Print and shaded views of the part. All mm, measured from the part's lowest x, y and z. Give positions to 0.01 mm unless a question says otherwise; leave off trailing zeros. Loops run counter-clockwise (first coordinate to the right, second up) from the corner with the lowest first, then second, coordinate; pieces in that order, holes last. Notation, with made-up numbers: (13.25, 68.5) - (55.25, 68.5) arc R21 cw to (55.25, 80.5) - close; hole circle Ø11 at (3.25, 74). An arc over 180 degrees is marked (long way). Return JSON: item names as keys, results as strings.
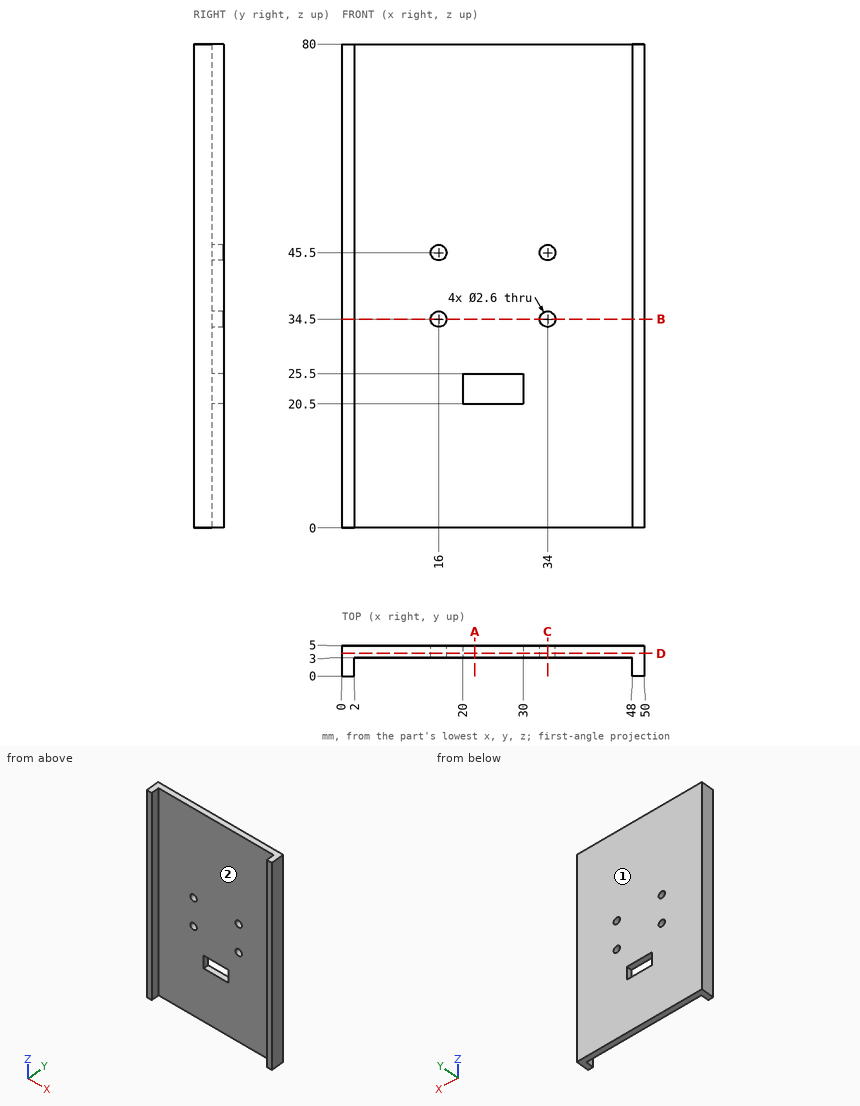
1. Cut at B-B, the plane z = 34.5. Write the cut outline in (x, y).
Values follow:
{"outline": "(0, 0) - (2, 0) - (2, 3) - (14.7, 3) - (14.7, 5) - (0, 5) - close; (17.3, 3) - (32.7, 3) - (32.7, 5) - (17.3, 5) - close; (35.3, 3) - (48, 3) - (48, 0) - (50, 0) - (50, 5) - (35.3, 5) - close"}
2. Cut at C-C, the plane x = 34. Write the cut outline in (y, z), plus the area to 3 significant figures.
Values follow:
{"outline": "(3, 0) - (5, 0) - (5, 33.2) - (3, 33.2) - close; (3, 35.8) - (5, 35.8) - (5, 44.2) - (3, 44.2) - close; (3, 46.8) - (5, 46.8) - (5, 80) - (3, 80) - close", "area": "150 mm²"}
3. Drill centre lines: probe 1 along Z at (x, y) = (34, 4.55); probe 2 along X at (y, z) = (4, 45.5); probe 3 along Z at (x, y) = (21, 4.3). Where is each one in solid material? Low to high.
Values follow:
{"probe 1": "z = 0 to 33.2, 35.8 to 44.2, 46.8 to 80", "probe 2": "x = 0 to 14.7, 17.3 to 32.7, 35.3 to 50", "probe 3": "z = 0 to 20.5, 25.5 to 80"}
4. Cut at D-D, the plane y = 3.75. Write the cut outline in (x, z).
Values follow:
{"outline": "(0, 0) - (50, 0) - (50, 80) - (0, 80) - close; hole circle Ø2.6 at (16, 34.5); hole circle Ø2.6 at (16, 45.5); hole (20, 20.5) - (30, 20.5) - (30, 25.5) - (20, 25.5) - close; hole circle Ø2.6 at (34, 34.5); hole circle Ø2.6 at (34, 45.5)"}
5. Cut at A-A, the plane x = 22. Write the cut outline in (y, z), plus the area to 3 significant figures.
Values follow:
{"outline": "(3, 0) - (5, 0) - (5, 20.5) - (3, 20.5) - close; (3, 25.5) - (5, 25.5) - (5, 80) - (3, 80) - close", "area": "150 mm²"}
6. Pull direction X, two halves, no side cores. Call the marked faces 1 and 2: +X half, -X half, draft (parallel to the pull), parting line (faces both ways), or undercut.
Values follow:
{"face 1": "draft", "face 2": "undercut"}
7. Drop flat-ended pins along their axis: P1, Ø0.6, axis at y = 4.5, z = 22, coming from the -X side; P2, Ø23, axis at x = 26.5, z = 52.5, coming from the -Y side. Give the stop position or say it passes through.
Values follow:
{"P1": "stops at x = 0", "P2": "stops at y = 3"}
